```python
from build123d import *

# Parameters (mm, degrees)
SKETCH1_W                = 98
SKETCH1_H                = 42
BOSS_EXTRUDE1_DEPTH      = 20
SKETCH2_W                = 70
SKETCH2_H                = 6
CUT_EXTRUDE1_DEPTH       = 68.564783726
SKETCH3_R                = 6
CUT_EXTRUDE2_DEPTH       = 14
BOSS_EXTRUDE2_DEPTH      = 7
BOSS_EXTRUDE2_DEPTH_BACK = 7
SKETCH4_W                = 42
SKETCH4_H                = 42
FILLET1_RADIUS           = 21
FILLET1_LENGTH           = 14
SKETCH5_R                = 10
CUT_EXTRUDE3_DEPTH       = 14


with BuildPart() as part:
    # Sketch1 → Boss-Extrude1 (new body)
    with BuildSketch(Plane(origin=(0, 0, 0), x_dir=(1, 0, 0), z_dir=(0, 1, 0))):
        Rectangle(SKETCH1_W, SKETCH1_H)
    extrude(amount=BOSS_EXTRUDE1_DEPTH)

    # Sketch2 → Cut-Extrude1 (cut, through all)
    with BuildSketch(Plane.XY.offset(21)):
        with Locations((0, 3)):
            Rectangle(SKETCH2_W, SKETCH2_H)
    extrude(amount=-CUT_EXTRUDE1_DEPTH, mode=Mode.SUBTRACT)

    # Sketch3 → Cut-Extrude2 (cut)
    with BuildSketch(Plane(origin=(0, 20, 0), x_dir=(1, 0, 0), z_dir=(0, 1, 0))):
        with Locations(Location((25, 0, 0), (0, 0, 270))):
            Circle(SKETCH3_R)
        with Locations(Location((-25, 0, 0), (0, 0, 270))):
            Circle(SKETCH3_R)
    extrude(amount=-CUT_EXTRUDE2_DEPTH, mode=Mode.SUBTRACT)

    # Sketch4 → Boss-Extrude2 (add, two sides: drawn at the far end of the back side and taken through both)
    with BuildSketch(Plane(origin=(0, 0, 0), x_dir=(0, 0, -1), z_dir=(1, 0, 0)).offset(-BOSS_EXTRUDE2_DEPTH_BACK)):
        with Locations((0, 41)):
            Rectangle(SKETCH4_W, SKETCH4_H)
    extrude(amount=BOSS_EXTRUDE2_DEPTH + BOSS_EXTRUDE2_DEPTH_BACK)

    # Fillet1: full round fillet: the end face becomes a half cylinder, R = half its width
    fillet1_face = Plane((0, 62, 0), x_dir=(1, 0, 0), z_dir=(0, 1, 0))  # on the end face: x along it, z out of the body
    fillet1_slab = fillet1_face.offset(-FILLET1_RADIUS / 2) * Box(FILLET1_LENGTH, 2 * FILLET1_RADIUS, FILLET1_RADIUS, mode=Mode.PRIVATE)  # the body's end, R deep
    fillet1_round = Plane((0, 41, 0), x_dir=(0, 1, 0), z_dir=(1, 0, 0)) * Cylinder(FILLET1_RADIUS, FILLET1_LENGTH, mode=Mode.PRIVATE)  # its axis R under the face
    add(fillet1_slab - fillet1_round, mode=Mode.SUBTRACT)

    # Sketch5 → Cut-Extrude3 (cut)
    with BuildSketch(Plane(origin=(7, 0, 0), x_dir=(0, 0, -1), z_dir=(1, 0, 0))):
        with Locations((0, 41)):
            Circle(SKETCH5_R)
    extrude(amount=-CUT_EXTRUDE3_DEPTH, mode=Mode.SUBTRACT)


solid = part.part
```
Input: part model. Units: mm. Frame: model coordinates. A direction names the side the tool comes from. Round coordinates to 2 decimals unless told otherwise and drop trailing zeros. Order: outer loops, then holes, each group sorted by start corner. A loop starts at its lowest first (then second) coordinate and runs counter-clockwise, first axis right, second up. Notation, with made-up numbers: (19.5, -28) - (27.5, -28) arc R13 cw to (27.5, -22) - close; hole circle Ø4 at (-3.75, 2). An arc over 180 degrees is marked (long way). Answer in a Markdown table with one row per item.
Item 1: Pin query (flat end, axial travel): pin 1 (21 mm diameter, centred on x = 1.5, z = 3, fed in from -Y); pin 2 (12.5 mm diameter, centred on x = -18.5, z = -8.5, fed in from +Y); pin 3 (6 mm diameter, centred on y = 55, z = 6.5, fed in from +X). Return the tip coordinate at first contact, or that it passes through.
Model answer:
| item | result |
|---|---|
| pin 1 | stops at y = 6 |
| pin 2 | stops at y = 20 |
| pin 3 | stops at x = 7 |
Item 2: Section query B-B (x = 25). Return the cut outline in (y, z).
Model answer:
| item | result |
|---|---|
| outline | (6, -21) - (20, -21) - (20, -6) - (6, -6) - close; (6, 6) - (20, 6) - (20, 21) - (6, 21) - close |
Item 3: Section query A-A (z = 0). Return the cut outline in (x, y), then the cut area to 3 significant figures.
Model answer:
| item | result |
|---|---|
| outline | (-49, 0) - (-35, 0) - (-35, 6) - (-31, 6) - (-31, 20) - (-49, 20) - close; (-19, 6) - (19, 6) - (19, 20) - (7, 20) - (7, 31) - (-7, 31) - (-7, 20) - (-19, 20) - close; (-7, 51) - (7, 51) - (7, 62) - (-7, 62) - close; (31, 6) - (35, 6) - (35, 0) - (49, 0) - (49, 20) - (31, 20) - close |
| area | 1,510 mm² |
Item 4: Section query C-C (y = 4). Return the cut outline in (x, z), then the cut area to 3 significant figures.
Model answer:
| item | result |
|---|---|
| outline | (-49, -21) - (-35, -21) - (-35, 21) - (-49, 21) - close; (35, -21) - (49, -21) - (49, 21) - (35, 21) - close |
| area | 1,180 mm² |
Item 5: Mould query, pull axis X, two halves, no side actions, for faces 1 (the flat face through (35, 3, 0)), 2 (the flat face through (7, 32, 5)), 3 (the flat face through (32, 20, 0)). Classes: released by +X, released by -X, zero draft, split by the parting line, or undercut.
Model answer:
| item | result |
|---|---|
| face 1 | undercut |
| face 2 | released by +X |
| face 3 | zero draft |
Item 6: Line query: line 1 (X direction, y = 12.5, z = 0.5); line 2 (X direction, y = 5, z = -7); line 3 (Z direction, x = 3, y = 33). Output: solid intervals per line, ascending.
Model answer:
| item | result |
|---|---|
| line 1 | x = -49 to -30.98, -19.02 to 19.02, 30.98 to 49 |
| line 2 | x = -49 to -35, 35 to 49 |
| line 3 | z = -21 to -6, 6 to 21 |
Item 7: Section query D-D (y = 17.5). Return the cut outline in (x, z).
Model answer:
| item | result |
|---|---|
| outline | (-49, -21) - (49, -21) - (49, 21) - (-49, 21) - close; hole circle Ø12 at (-25, 0); hole circle Ø12 at (25, 0) |
Item 8: Reachability of faces 4 (the flat face through (-1, 11, 21)), 5 (the flat face through (-7, 32, 5)), 6 (the flat face through (0, 6, 0)) from +Z, -Z, +X, -X, +Y, -Y: full face, straight path, thin tool, end or side. Return the list, or none.
Model answer:
| item | result |
|---|---|
| face 4 | +Z, +X, -X, +Y, -Y |
| face 5 | +Z, -Z, -X, +Y |
| face 6 | +Z, -Z, -Y |
